Here's how the part is built. I have some questions about the finished solid (model axes, mm). Coordinates: 2 decimals unless noted, no trailing zeros. Write each loop counter-clockwise with the first axis right and the second up, starting at its lowest first coordinate (ties: lowest second). Pieces come first, ordered by that corner, then holes. Notation, with made-up numbers: M 65.5,-39 L 119.5,-39 A21 ccw 119.5,-15 Z; hole C 48.25,86 d3. An arc over 180 degrees is marked long. Use one line per item in the form item = value. Start each with the question number.
1. I want a section at B-B, the plane x = -20. List the corners of the cut face in (y, z) for me.
2. Please list where these lines run through material, in increasing order: line 1 along Y through (x, z) = (-9, 20.75) (3 decimals); line 2 along Y through (x, z) = (0, 18.25); line 3 along X through (y, z) = (30, 22.5). Write a range as [from, to].
3. I want a section at A-A, the plane y = 11. List the corners of the cut face in (x, z) for me.
4. I'm going to push flat-ended pins straight in: pin 1 Ø10 at (x, z) = (-38.5, 10) entering from +Y; pin 2 Ø3 at (y, z) = (0.5, 4.5) entering from +X; pin 3 Ø5 at (x, z) = (-35.5, 22) entering from +Y. Where does each tip first touch, or does it pass through?
5. Thinking about a two-plate mould opening in Y: for faces 1 (the face through (-7.058, -31.786, 12.522)), 2 (the face through (-22.1, 24.3, 25.4)), 3 (the face through (46.11, 26.15, 12.52)), 4 (the face through (45.7, -26.86, 12.52)), which applies, released by +Y, released by -Y, zero draft, split by the parting line, or undercut?
6. I want a section at C-C, the plane z = 21. List the corners of the cut face in (x, y) for me.
from build123d import *

# Parameters (mm, degrees)
F0_R     = 32.560597
F1_DEPTH = 25.4
F2_SIZE2 = 5.08
F2_SIZE  = 5.08


with BuildPart() as f1:
    # F0 (on Top) → F1 (new body)
    with BuildSketch(Plane.XY):
        Polygon((-0.49722, -55.545455), (47.855165, -28.203333), (48.352385, 27.342122), (0.49722, 55.545455), (-47.855165, 28.203333), (-48.352385, -27.342122), align=None)
        Circle(F0_R, mode=Mode.SUBTRACT)
    extrude(amount=F1_DEPTH)

    # F2
    f2_edges = [f1.edges().sort_by_distance(p)[0] for p in [
        (-48.352385, -27.342122, 12.7),
        (-47.855165, 28.203333, 12.7),
        (-0.49722, -55.545455, 12.7),
        (0.49722, 55.545455, 12.7),
        (48.352385, 27.342122, 12.7),
        (47.855165, -28.203333, 12.7),
    ]]
    chamfer(f2_edges, length=F2_SIZE, length2=F2_SIZE2)


solid = f1.part
Answer list:
q1.outline = M -44.05,0 L -25.69,0 L -25.69,25.4 L -44.05,25.4 Z; M 25.69,0 L 43.95,0 L 43.95,25.4 L 25.69,25.4 Z
q2.line_1 = [-50.534, -31.292], [31.292, 50.175]
q2.line_2 = [-53.01, -32.56], [32.56, 53.01]
q2.line_3 = [-43.85, -12.66], [12.66, 43.84]
q3.outline = M -48.01,0 L -30.65,0 L -30.65,25.4 L -48.01,25.4 Z; M 30.65,0 L 48.21,0 L 48.21,25.4 L 30.65,25.4 Z
q4.pin_1 = 36.32
q4.pin_2 = 48.13
q4.pin_3 = 36.6
q5.face_1 = undercut
q5.face_2 = zero draft
q5.face_3 = released by +Y
q5.face_4 = released by -Y
q6.outline = M -48.31,-22.26 L -43.98,-29.92 L -4.87,-52.97 L 3.92,-53.04 L 43.43,-30.7 L 47.9,-23.12 L 48.31,22.26 L 43.98,29.92 L 4.87,52.97 L -3.92,53.04 L -43.43,30.7 L -47.9,23.12 Z; hole C 0,0 d65.12
